from build123d import *

# Parameters (mm, degrees)
IZIM1_W                     = 35
IZIM1_H                     = 50
IZIM1_W_2                   = 0.6
IZIM1_H_2                   = 0.6
IZIM1_W_3                   = 0.65
IZIM1_H_3                   = 0.45
Y_KSEKLIK_EKSTR_ZYON1_DEPTH = 2
IZIM2_W                     = 0.65
IZIM2_H                     = 50
Y_KSEKLIK_EKSTR_ZYON2_DEPTH = 10
IZIM3_W                     = 10
IZIM3_H                     = 1.2
Y_KSEKLIK_EKSTR_ZYON3_DEPTH = 17.175
IZIM4_W                     = 7.5
IZIM4_H                     = 0.8
KES_EKSTR_ZYON1_DEPTH       = 10
KES_EKSTR_ZYON2_REACH       = 49.011
IZIM5_RX                    = 3.75
IZIM5_RY                    = 3.75


with BuildPart() as part:
    # Çizim1 → Yükseklik-Ekstrüzyon1 (new body)
    with BuildSketch(Plane.XY):
        with Locations((17.5, 25)):
            Rectangle(IZIM1_W, IZIM1_H)
        with Locations((8.3, 5.703429896)):
            Rectangle(IZIM1_W_2, IZIM1_H_2, mode=Mode.SUBTRACT)
        with Locations((10.84, 5.703429896)):
            Rectangle(IZIM1_W_2, IZIM1_H_2, mode=Mode.SUBTRACT)
        with Locations((27, 5.375)):
            Rectangle(IZIM1_W_3, IZIM1_H_3, mode=Mode.SUBTRACT)
        with Locations((24.5, 5.375)):
            Rectangle(IZIM1_W_3, IZIM1_H_3, mode=Mode.SUBTRACT)
    extrude(amount=Y_KSEKLIK_EKSTR_ZYON1_DEPTH)

    # Çizim2 → Yükseklik-Ekstrüzyon2 (add)
    with BuildSketch(Plane.XY.offset(2)):
        with Locations((17.5, 25)):
            Rectangle(IZIM2_W, IZIM2_H)
    extrude(amount=Y_KSEKLIK_EKSTR_ZYON2_DEPTH)

    # Çizim3 → Yükseklik-Ekstrüzyon3 (add, through all)
    with BuildSketch(Plane.ZY.offset(-17.175)):
        with Locations((7, 21.6)):
            Rectangle(IZIM3_W, IZIM3_H)
    extrude(amount=Y_KSEKLIK_EKSTR_ZYON3_DEPTH)

    # Çizim4 → Kes-Ekstrüzyon1 (cut)
    with BuildSketch(Plane.XY.offset(12)):
        with Locations((9.57, 21.6)):
            Rectangle(IZIM4_W, IZIM4_H)
    extrude(amount=-KES_EKSTR_ZYON1_DEPTH, mode=Mode.SUBTRACT)

    # Çizim5 → Kes-Ekstrüzyon2 (cut, up to next)
    with BuildSketch(Plane.XZ.offset(-21), mode=Mode.PRIVATE) as kes_ekstr_zyon2_sk1:
        with Locations(Location((9.224839589, 6), (0, 0, 180))):
            Ellipse(IZIM5_RX, IZIM5_RY)
    kes_ekstr_zyon2_tool1 = extrude(kes_ekstr_zyon2_sk1.sketch, amount=-KES_EKSTR_ZYON2_REACH, mode=Mode.PRIVATE) & part.part
    add(kes_ekstr_zyon2_tool1.solids().sort_by_distance((9.22484, 21, 6))[0], mode=Mode.SUBTRACT)


solid = part.part
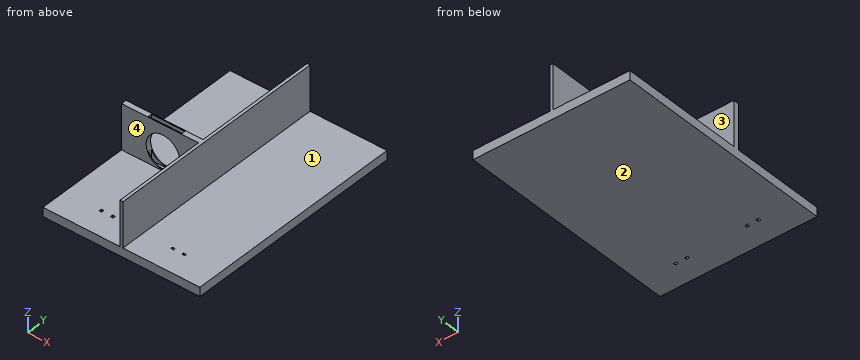
Model file for the job. Use its own axes, mm. Face numbers are marked on the shaded views. A direction names the side the tool comes from. Round coordinates to 2 decimals unless told otherwise and drop trailing zeros. Order: outer loops, then holes, each group sorted by start corner. A loop starts at its lowest first (then second) coordinate and runs counter-clockwise, first axis right, second up. Notation, with made-up numbers: M 8,70.5 L 25,70.5 A15 cw 25,75.5 Z; hole C -25,88 d1. An arc over 180 degrees is marked long. Write each question's results on one line, items separated by ' | '. Start each with the question number.
(1) Which spindle directions (+Z, -Z, +X, -X, +Y, -Y) get a long thin tool onto all of the face, cutting with end or side? Do the marked faces 1, 2, 3 and 4. Say none if no direction does.
(2) Saw through at C-C, the plane y = 24.5. Give the cut face in (x, z) (3 decimals).
(3) Saw through at D-D, the plane x = 9.5. State how many separate pieces and enclosed holes the cut face has, then the cut area to 3 significant figures.
(4) Saw through at B-B, the plane x = 16.5. Give the cut face in (y, z), then the cut area to 3 significant figures.
(5) Saw through at A-A, the plane z = 11. Give the cut face in (x, y) (3 decimals).
(6) Probe probe 1 along Y at (x, z) = (10.5, 10.5); probe 2 along Y at (x, z) = (5, 9); probe 3 along Z at (x, y) = (18.5, 14). List the from-to ranges inside material, lowest first. Write a range as from..to.
(7) Drop flat-ended pins along their axis: pin 1 (1.5 mm diameter, centred on x = 7.5, y = 39.5, fed in from +Z); pin 2 (5 mm diameter, centred on x = 11.5, z = 6.5, fed in from -Y); pin 3 (4 mm diameter, centred on y = 14, z = 5, fed in from -X) (3 decimals); pin 4 (4 mm diameter, centred on x = 26.5, z = 5.5, fed in from -Y). Give the stop position or say it passes through.
Established:
1) face 1: +Z, +X, +Y, -Y | face 2: -Z, +X, -X, +Y, -Y | face 3: +Z, -X, +Y | face 4: +Z, -X, -Y
2) outline: M 0,0 L 35,0 L 35,2 L 17.825,2 L 17.825,12 L 17.175,12 L 17.175,2 L 0,2 Z
3) separate pieces: 3 | enclosed holes: 0 | area: 101 mm^2
4) outline: M 0,0 L 50,0 L 50,2 L 22.2,2 L 22.2,12 L 21,12 L 21,2 L 0,2 Z | area: 112 mm^2
5) outline: M 0,21 L 17.175,21 L 17.175,0 L 17.825,0 L 17.825,50 L 17.175,50 L 17.175,22.2 L 0,22.2 Z; hole M 5.82,21.2 L 13.32,21.2 L 13.32,22 L 5.82,22 Z
6) probe 1: y = 21..21.2, 22..22.2 | probe 2: y = 21..22.2 | probe 3: z = 0..2
7) pin 1: stops at z = 2 | pin 2: stops at y = 21 | pin 3: stops at x = 17.175 | pin 4: passes through
